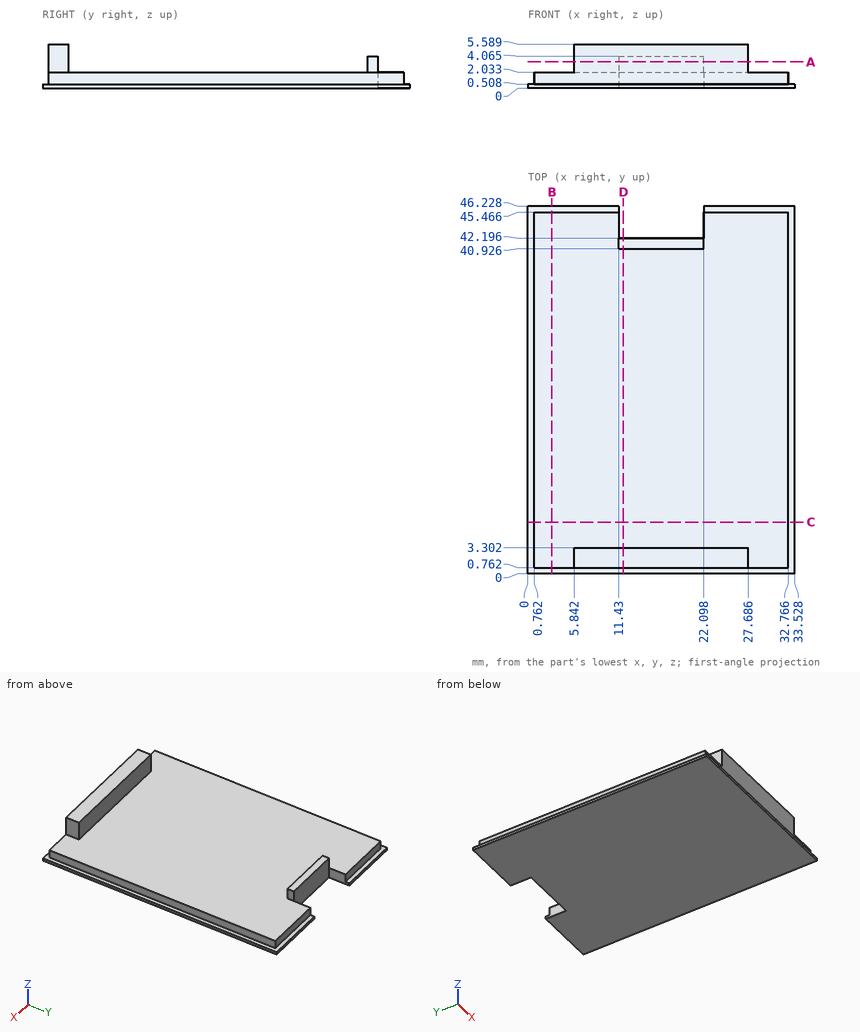
Study the drawing (mm; zero at the part's minimum x, y, z) and answer. Give positions to 0.01 mm unless a question says otherwise; leave off trailing zeros. Order: outer loops, then holes, each group sorted by start corner. A loop starts at its lowest first (then second) coordinate and runs counter-clockwise, first axis right, second up. Notation, with made-up numbers: (-15.5, 70) - (-5.5, 70) arc R11 ccw to (-5.5, 77) - close; hole circle Ø11 at (-26, 76). An arc over 180 degrees is marked (long way). Answer as CSV lines item,"result". Start each with the question number.
Q1. The part is cut by section A-A (z = 3.35). Write down the section's boundary in (x, y).
Q2. Given pin 1 Ø8 at (x, y) = (27, 24) entering from +Z; pin 2 Ø1.4 at (y, z) = (41.5, 3) entering from +X; pin 3 Ø0.8 at (y, z) = (1.5, 4) entering from -X; pin 4 Ø2 at (x, z) = (9.5, 1) entering from -Y, each flat-ended and moving along its own axis, determine where each tip first touches the part or whether it passes through.
Q3. The part is cut by section C-C (y = 6.5). Write down the section's boundary in (x, z).
Q4. The part is cut by section D-D (x = 12). Write down the section's boundary in (y, z) (1 decimal).
Q5. Find the intervals of material crossed by L1, parallel to Z at x = 4, y = 20.5; L2, parallel to Y at x = 25.5, z = 4.95; L3, parallel to X at y = 28, z = 1.2, in increasing order. Write a range as [from, to].
Q6. The part is cut by section B-B (x = 3). Write down the section's boundary in (y, z).
Check result:
1,outline,"(5.84, 0.76) - (27.69, 0.76) - (27.69, 3.3) - (5.84, 3.3) - close; (11.43, 40.93) - (22.1, 40.93) - (22.1, 42.2) - (11.43, 42.2) - close"
2,pin 1,"stops at z = 2.03"
2,pin 2,"stops at x = 22.1"
2,pin 3,"stops at x = 5.84"
2,pin 4,"stops at y = 0"
3,outline,"(0, 0) - (33.53, 0) - (33.53, 0.51) - (32.77, 0.51) - (32.77, 2.03) - (0.76, 2.03) - (0.76, 0.51) - (0, 0.51) - close"
4,outline,"(0, 0) - (42.2, 0) - (42.2, 4.1) - (40.9, 4.1) - (40.9, 2) - (3.3, 2) - (3.3, 5.6) - (0.8, 5.6) - (0.8, 0.5) - (0, 0.5) - close"
5,L1,"z = [0, 2.03]"
5,L2,"y = [0.76, 3.3]"
5,L3,"x = [0.76, 32.77]"
6,outline,"(0, 0) - (46.23, 0) - (46.23, 0.51) - (45.47, 0.51) - (45.47, 2.03) - (0.76, 2.03) - (0.76, 0.51) - (0, 0.51) - close"
